Build history of the part. All positions in model axes, mm. Round coordinates to 2 decimals unless told otherwise and drop trailing zeros. Write each loop counter-clockwise with the first axis right and the second up, starting at its lowest first coordinate (ties: lowest second). Pieces come first, ordered by that corner, then holes. Notation, with made-up numbers: (-17, 52) -> (26, 52) arc R18 cw to (26, 77) -> close; hole circle Ø3 at (67.25, -18). An arc over 180 degrees is marked (long way). Answer in a Markdown table with one row per item.
```python
from build123d import *

# Parameters (mm, degrees)
EXTRUDE_START         = -150
EXTRUDE_1_DEPTH       = 2855.29255553
EXTRUDE_START_2       = -2356
EXTRUDE_1_2_OUTLINE_W = 61
EXTRUDE_1_2_OUTLINE_H = 53
EXTRUDE_1_2_DEPTH     = 25.647922242
SKETCH_2_R            = 9.5
CUT_EXTRUDE_1_DEPTH   = 2706.870065433


with BuildPart() as part:
    # Бобышка-Вытянуть1: read off the stored shape, not the designer's step
    # Бобышка-Вытянуть1 outline → Бобышка-Вытянуть1 (new body)
    with BuildSketch(Plane(origin=(0, 0, 0), x_dir=(1, 0, 0), z_dir=(0, 1, 0)).offset(EXTRUDE_START)):
        with BuildLine():
            Line((-25, 22), (-25, -22))
            ThreePointArc((-25, -22), (-24.121320344, -24.121320344), (-22, -25))
            Line((-22, -25), (22, -25))
            ThreePointArc((22, -25), (24.121320344, -24.121320344), (25, -22))
            Line((25, -22), (25, 22))
            ThreePointArc((25, 22), (24.121320344, 24.121320344), (22, 25))
            Line((22, 25), (-22, 25))
            ThreePointArc((-22, 25), (-24.121320344, 24.121320344), (-25, 22))
        make_face()
        with BuildLine():
            ThreePointArc((-20, -22), (-21.414213562, -21.414213562), (-22, -20))
            Line((-22, -20), (-22, 20))
            ThreePointArc((-22, 20), (-21.414213562, 21.414213562), (-20, 22))
            Line((-20, 22), (20, 22))
            ThreePointArc((20, 22), (21.414213562, 21.414213562), (22, 20))
            Line((22, 20), (22, -20))
            ThreePointArc((22, -20), (21.414213562, -21.414213562), (20, -22))
            Line((20, -22), (-20, -22))
        make_face(mode=Mode.SUBTRACT)
    extrude(amount=EXTRUDE_1_DEPTH)

    # Extrude 1 2 outline → Extrude 1 2 (cut)
    with BuildSketch(Plane(origin=(0, 0, 0), x_dir=(0.8660254037844386, 0.4999999999999999, 0), z_dir=(0.4999999999999999, -0.8660254037844388, 0)).offset(EXTRUDE_START_2)):
        with Locations((1345.5, -0.5)):
            Rectangle(EXTRUDE_1_2_OUTLINE_W, EXTRUDE_1_2_OUTLINE_H)
    extrude(amount=EXTRUDE_1_2_DEPTH, mode=Mode.SUBTRACT)

    # Эскиз2 → Вырез-Вытянуть1 (cut, through all)
    with BuildSketch(Plane(origin=(25, 0, 0), x_dir=(0, 0, -1), z_dir=(1, 0, 0))):
        with Locations((0, 50)):
            Circle(SKETCH_2_R)
    extrude(amount=-CUT_EXTRUDE_1_DEPTH, mode=Mode.SUBTRACT)


solid = part.part
```
Q1. Saw through at A-A on y = 1187.5. Write the cut outline in (x, z).
A:
| item | result |
|---|---|
| outline | (-25, -22) arc R3 ccw to (-22, -25) -> (22, -25) arc R3 ccw to (25, -22) -> (25, 22) arc R3 ccw to (22, 25) -> (-22, 25) arc R3 ccw to (-25, 22) -> close; hole (-22, -20) arc R2 ccw to (-20, -22) -> (20, -22) arc R2 ccw to (22, -20) -> (22, 20) arc R2 ccw to (20, 22) -> (-20, 22) arc R2 ccw to (-22, 20) -> close |
Q2. Saw through at B-B on z = 0. Write the cut outline in (x, y).
A:
| item | result |
|---|---|
| outline | (-25, -150) -> (-22, -150) -> (-22, 40.5) -> (-25, 40.5) -> close; (-25, 59.5) -> (-22, 59.5) -> (-22, 2678.16) -> (-25, 2676.43) -> close; (22, -150) -> (25, -150) -> (25, 40.5) -> (22, 40.5) -> close; (22, 59.5) -> (25, 59.5) -> (25, 2705.29) -> (22, 2703.56) -> close |
Q3. Saw through at C-C on x = -1.5. Write the cut outline in (y, z), plus the area to 3 significant figures.
A:
| item | result |
|---|---|
| outline | (-150, -25) -> (2689.99, -25) -> (2689.99, -22) -> (-150, -22) -> close; (-150, 22) -> (2689.99, 22) -> (2689.99, 25) -> (-150, 25) -> close |
| area | 17,000 mm² |
Q4. Wall check: line 1 (X direction, y = 807, z = 7.5); line 2 (X direction, y = 928, z = 20.5). Give the ranges that are in metal, low to high. Write a range as [from, to].
A:
| item | result |
|---|---|
| line 1 | [-25, -22], [22, 25] |
| line 2 | [-25, -21.94], [21.94, 25] |
